CAD build for the part. Positions are in the model's coordinates, mm. Face numbers are marked on the shaded views. A direction names the side the tool comes from. Round coordinates to 2 decimals unless told otherwise and drop trailing zeros. Loops run counter-clockwise (first coordinate to the right, second up) from the corner with the lowest first, then second, coordinate; pieces in that order, holes last.
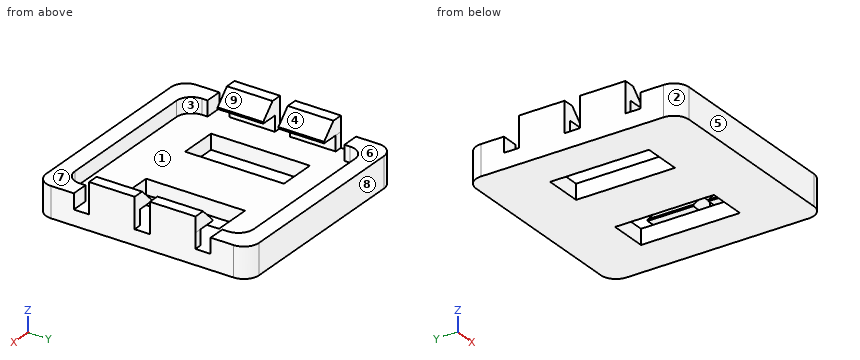
from build123d import *

# Parameters (mm, degrees)
BOSS_EXTRU_1_DEPTH           = 4
ENL_V_MAT_EXTRU_1_DEPTH      = 2
ESQUISSE3_W                  = 5
ESQUISSE3_H                  = 13
ENL_V_MAT_EXTRU_2_DEPTH      = 20.899748742
ESQUISSE4_W                  = 3.25
ESQUISSE4_H                  = 5.994249795
ESQUISSE4_H_2                = 6.005750205
BOSS_EXTRU_2_DEPTH           = 2
CHANFREIN3_SIZE              = 1.8
CHANFREIN3_OF_SYM_TRIE1_SIZE = 1.8


with BuildPart() as part:
    # Esquisse1 → Boss.-Extru.1 (new body)
    with BuildSketch(Plane.XY):
        with BuildLine():
            Line((12, -14), (-12, -14))
            ThreePointArc((-12, -14), (-13.414213562, -13.414213562), (-14, -12))
            Line((-14, -12), (-14, 12))
            ThreePointArc((-14, 12), (-13.414213562, 13.414213562), (-12, 14))
            Line((-12, 14), (12, 14))
            ThreePointArc((12, 14), (13.414213562, 13.414213562), (14, 12))
            Line((14, 12), (14, -12))
            ThreePointArc((14, -12), (13.414213562, -13.414213562), (12, -14))
        make_face()
    extrude(amount=BOSS_EXTRU_1_DEPTH)

    # Esquisse2 → Enlèv. mat.-Extru.1 (cut)
    with BuildSketch(Plane.XY.offset(4)):
        with BuildLine():
            Line((-9.75, -11.75), (9.75, -11.75))
            ThreePointArc((9.75, -11.75), (11.164213562, -11.164213562), (11.75, -9.75))
            Line((11.75, -9.75), (11.75, -9))
            Line((11.75, -9), (14, -9))
            Line((14, -9), (14, -7))
            Line((14, -7), (13, -7))
            Line((13, -7), (13, -1.005750205))
            Line((13, -1.005750205), (14, -1.005750205))
            Line((14, -1.005750205), (14, 0.994249795))
            Line((14, 0.994249795), (13, 0.994249795))
            Line((13, 0.994249795), (13, 6.988499589))
            Line((13, 6.988499589), (14, 6.988499589))
            Line((14, 6.988499589), (14, 8.988499589))
            Line((14, 8.988499589), (11.75, 8.988499589))
            Line((11.75, 8.988499589), (11.75, 9.75))
            ThreePointArc((11.75, 9.75), (11.164213562, 11.164213562), (9.75, 11.75))
            Line((9.75, 11.75), (-9.75, 11.75))
            ThreePointArc((-9.75, 11.75), (-11.164213562, 11.164213562), (-11.75, 9.75))
            Line((-11.75, 9.75), (-11.75, 8.988499589))
            Line((-11.75, 8.988499589), (-14, 8.988499589))
            Line((-14, 8.988499589), (-14, 6.988499589))
            Line((-14, 6.988499589), (-13, 6.988499589))
            Line((-13, 6.988499589), (-13, 0.994249795))
            Line((-13, 0.994249795), (-14, 0.994249795))
            Line((-14, 0.994249795), (-14, -1.005750205))
            Line((-14, -1.005750205), (-13, -1.005750205))
            Line((-13, -1.005750205), (-13, -7))
            Line((-13, -7), (-14, -7))
            Line((-14, -7), (-14, -9))
            Line((-14, -9), (-11.75, -9))
            Line((-11.75, -9), (-11.75, -9.75))
            ThreePointArc((-11.75, -9.75), (-11.164213562, -11.164213562), (-9.75, -11.75))
        make_face()
    extrude(amount=-ENL_V_MAT_EXTRU_1_DEPTH, mode=Mode.SUBTRACT)

    # Esquisse3 → Enlèv. mat.-Extru.2 (cut, through all)
    with BuildSketch(Plane.XY.offset(2)):
        with Locations((-6.25, 0)):
            Rectangle(ESQUISSE3_W, ESQUISSE3_H)
        with Locations((6.25, 0)):
            Rectangle(ESQUISSE3_W, ESQUISSE3_H)
    extrude(amount=-ENL_V_MAT_EXTRU_2_DEPTH, mode=Mode.SUBTRACT)

    # Esquisse4 → Boss.-Extru.2 (add)
    with BuildSketch(Plane.XY.offset(4)):
        with Locations((-12.375, -4.002875103)):
            Rectangle(ESQUISSE4_W, ESQUISSE4_H)
        with Locations((-12.375, 3.997124897)):
            Rectangle(ESQUISSE4_W, ESQUISSE4_H_2)
    boss_extru_2 = extrude(amount=BOSS_EXTRU_2_DEPTH)

    # Chanfrein3
    chanfrein3_edges = [part.edges().sort_by_distance(p)[0] for p in [
        (-10.75, 3.997124897, 6),
        (-10.75, -4.002875103, 6),
    ]]
    chamfer(chanfrein3_edges, length=CHANFREIN3_SIZE)

    # Symétrie1: Boss.-Extru.2 across plane
    add(boss_extru_2.mirror(Plane(origin=(0, 0, 0), x_dir=(0, 0, 1), z_dir=(1, 0, 0))))

    # Chanfrein3 of Symétrie1
    chanfrein3_of_sym_trie1_edges = [part.edges().sort_by_distance(p)[0] for p in [
        (10.75, 3.997124897, 6),
        (10.75, -4.002875103, 6),
    ]]
    chamfer(chanfrein3_of_sym_trie1_edges, length=CHANFREIN3_OF_SYM_TRIE1_SIZE)


solid = part.part
Item 1: Cut at C-C (y = 5.5). List the corners of the cut face in (x, z), plus the area to 3 significant figures.
Verdict:
outline: (-14, 0) - (-8.75, 0) - (-8.75, 2) - (-13, 2) - (-13, 4) - (-10.75, 4) - (-10.75, 4.2) - (-12.55, 6) - (-14, 6) - close; (-3.75, 0) - (3.75, 0) - (3.75, 2) - (-3.75, 2) - close; (8.75, 0) - (14, 0) - (14, 6) - (12.55, 6) - (10.75, 4.2) - (10.75, 4) - (13, 4) - (13, 2) - (8.75, 2) - close
area: 49.8 mm2
Item 2: Cut at A-A (z = 4.95). List the corners of the cut face in (x, y).
Verdict:
outline: (-14, -7) - (-11.5, -7) - (-11.5, -1.01) - (-14, -1.01) - close; (-14, 0.99) - (-11.5, 0.99) - (-11.5, 7) - (-14, 7) - close; (11.5, -7) - (14, -7) - (14, -1.01) - (11.5, -1.01) - close; (11.5, 0.99) - (14, 0.99) - (14, 7) - (11.5, 7) - close
Item 3: Cut at B-B (x = -7). List the corners of the cut face in (y, z).
Verdict:
outline: (-14, 0) - (-6.5, 0) - (-6.5, 2) - (-11.75, 2) - (-11.75, 4) - (-14, 4) - close; (6.5, 0) - (14, 0) - (14, 4) - (11.75, 4) - (11.75, 2) - (6.5, 2) - close
Item 4: 3-axis set-ups, long thin cutter, end or side, ignore diameter. For the marked faces 5, 6, 7, 8 and 9: which of +Z, -Z, +X, -X, +Y, -Y reach the whole face in a straight line?
Verdict:
face 5: +Z, -Z, +X, -X, -Y
face 6: +Z, +X, -X, +Y
face 7: +Z, +X, -X, -Y
face 8: +Z, -Z, +X, -X, +Y
face 9: +Z, +Y, -Y
Item 5: Cut at D-D (z = 0.9). List the corners of the cut face in (x, y), plus the area to 3 significant figures.
Verdict:
outline: (-14, -12) arc R2 ccw to (-12, -14) - (12, -14) arc R2 ccw to (14, -12) - (14, 12) arc R2 ccw to (12, 14) - (-12, 14) arc R2 ccw to (-14, 12) - close; hole (-8.75, -6.5) - (-3.75, -6.5) - (-3.75, 6.5) - (-8.75, 6.5) - close; hole (3.75, -6.5) - (8.75, -6.5) - (8.75, 6.5) - (3.75, 6.5) - close
area: 651 mm2
Item 6: Flat gauge pins, fed straight in: P1, Ø10, axis at x = 0.5, y = -6.5, coming from the +Z side; P2, Ø1.5, axis at x = -1.5, y = 11.5, coming from the +Z side; P3, Ø0.6, axis at x = -12, z = 5, coming from the +Y side. Where does each tip first touch, or does it go through?
Verdict:
P1: stops at z = 2
P2: stops at z = 4
P3: stops at y = 7
Item 7: Wall check: L1, parallel to X at y = -4, z = 0.35; L2, parallel to Y at x = 6.5, z = 3.2; L3, parallel to Y at x = 4.75, z = 0.95. Give the ranges that are in metal, low to high.
Verdict:
L1: x = -14 to -8.75, -3.75 to 3.75, 8.75 to 14
L2: y = -14 to -11.75, 11.75 to 14
L3: y = -14 to -6.5, 6.5 to 14
Item 8: Mould opens along Y. For the marked faces 1, 2, 3 and 4 say: released by +Y, released by -Y, zero draft, split by the parting line, or undercut.
Verdict:
face 1: undercut
face 2: released by -Y
face 3: undercut
face 4: zero draft
